```python
from build123d import *

# Parameters (mm, degrees)
SALIENTE_EXTRUIR1_DEPTH = 3
CORTAR_EXTRUIR1_DEPTH   = 3
CROQUIS3_R              = 1.5
CORTAR_EXTRUIR2_DEPTH   = 135.383778783
CROQUIS5_R              = 2
CORTAR_EXTRUIR3_DEPTH   = 135.383778783


with BuildPart() as part:
    # Croquis1 → Saliente-Extruir1 (new body)
    with BuildSketch(Plane.XY):
        Polygon((-39.350288425, -95), (39.350288425, -95), (95, -39.350288425), (95, 39.350288425), (39.350288425, 95), (-39.350288425, 95), (-95, 39.350288425), (-95, -39.350288425), align=None)
    extrude(amount=SALIENTE_EXTRUIR1_DEPTH)

    # Croquis2 → Cortar-Extruir1 (cut)
    with BuildSketch(Plane(origin=(0, 0, 0), x_dir=(-1, 0, 0), z_dir=(0, 0, -1))):
        Polygon((-69, -28.580735804), (-28.580735804, -69), (28.580735804, -69), (69, -28.580735804), (69, 28.580735804), (28.580735804, 69), (-28.580735804, 69), (-69, 28.580735804), align=None)
    extrude(amount=-CORTAR_EXTRUIR1_DEPTH, mode=Mode.SUBTRACT)

    # Croquis3 → Cortar-Extruir2 (cut, through all)
    with BuildSketch(Plane(origin=(0, 0, 0), x_dir=(-1, 0, 0), z_dir=(0, 0, -1))):
        with Locations((-19.5, 73)):
            Circle(CROQUIS3_R)
        with Locations((19.5, 73)):
            Circle(CROQUIS3_R)
        with Locations((-73, 19.5)):
            Circle(CROQUIS3_R)
        with Locations((-73, -19.5)):
            Circle(CROQUIS3_R)
        with Locations(Location((73, 19.5, 0), (0, 0, 180))):
            Circle(CROQUIS3_R)
        with Locations(Location((73, -19.5, 0), (0, 0, 180))):
            Circle(CROQUIS3_R)
    extrude(amount=-CORTAR_EXTRUIR2_DEPTH, mode=Mode.SUBTRACT)

    # Croquis5 → Cortar-Extruir3 (cut, through all)
    with BuildSketch(Plane.XY.offset(3)):
        with Locations((-42.892214845, 81.7)):
            Circle(CROQUIS5_R)
        with Locations((42.409372133, 81.9)):
            Circle(CROQUIS5_R)
        with Locations((-79, 29.894444303)):
            Circle(CROQUIS5_R)
        with Locations(Location((79, 29.894444303, 0), (0, 0, 180))):
            Circle(CROQUIS5_R)
    extrude(amount=-CORTAR_EXTRUIR3_DEPTH, mode=Mode.SUBTRACT)


solid = part.part
```
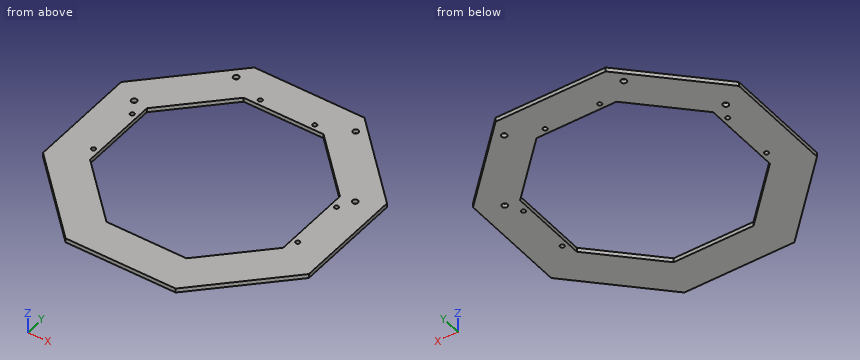
Input: part model. Units: mm. Frame: model coordinates. Give positions to 0.01 mm unless a question says otherwise; leave off trailing zeros. Order: outer loops, then holes, each group sorted by start corner. A loop starts at its lowest first (then second) coordinate and runs counter-clockwise, first axis right, second up.
1. Section A-A on y = 2. Return the cut outline in (x, z), and give its area (3 significant figures).
Derived:
outline: (-95, 0) - (-69, 0) - (-69, 3) - (-95, 3) - close; (69, 0) - (95, 0) - (95, 3) - (69, 3) - close
area: 156 mm2
2. Pin query (flat end, axial travel): pin 1 (1.5 mm diameter, centred on x = 54.5, z = 1, fed in from +Y). Return the tip coordinate at first contact, or that it passes through.
Derived:
pin 1: stops at y = 80.6
3. Section B-B on x = 52.5. Return the cut outline in (y, z), and give its area (3 significant figures).
Derived:
outline: (-81.85, 0) - (-45.08, 0) - (-45.08, 3) - (-81.85, 3) - close; (45.08, 0) - (81.85, 0) - (81.85, 3) - (45.08, 3) - close
area: 221 mm2
4. Material intervals for L1, parallel to X at y = -11.5, z = 0.95; L2, parallel to Y at x = -73, z = 1.65, sorted ascending.
Derived:
L1: x = -95 to -69, 69 to 95
L2: y = -61.35 to -21, -18 to 18, 21 to 61.35
5. Section C-C on z = 1.75. Give the number of separate pieces and of enclosed holes in the cut face, and give its area (3 significant figures).
Derived:
separate pieces: 1
enclosed holes: 11
area: 14,000 mm2
